```python
from build123d import *

# Parameters (mm, degrees)
ESQUISSE1_R          = 10
ESQUISSE1_R_2        = 4
BASE_EXTRUSION_DEPTH = 4
ESQUISSE2_R          = 7
ESQUISSE2_R_2        = 4
BOSS_EXTRU_1_DEPTH   = 3
CHANFREIN3_SIZE      = 0.5


with BuildPart() as part:
    # Esquisse1 → Base-Extrusion (new body)
    with BuildSketch(Plane.XY):
        Circle(ESQUISSE1_R)
        Circle(ESQUISSE1_R_2, mode=Mode.SUBTRACT)
    extrude(amount=BASE_EXTRUSION_DEPTH)

    # Esquisse2 → Boss.-Extru.1 (add)
    with BuildSketch(Plane.XY.offset(4)):
        Circle(ESQUISSE2_R)
        Circle(ESQUISSE2_R_2, mode=Mode.SUBTRACT)
    extrude(amount=BOSS_EXTRU_1_DEPTH)

    # Chanfrein3
    chanfrein3_edges = [part.edges().sort_by_distance(p)[0] for p in [
        (-7, 0, 7),
        (-4, 0, 7),
        (-4, 0, 0),
    ]]
    chamfer(chanfrein3_edges, length=CHANFREIN3_SIZE)


solid = part.part
```
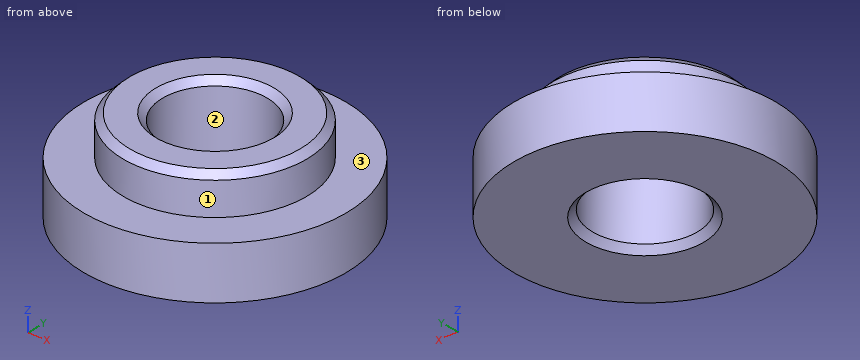
Geometry check sheet. Reference: the model listing, model coordinates, mm. Face numbers are marked on the shaded views. Coordinates: 2 decimals unless noted, no trailing zeros. Order: outer loops, then holes, each group sorted by start corner. A loop starts at its lowest first (then second) coordinate and runs counter-clockwise, first axis right, second up. Notation, with made-up numbers: (21, 11.25) - (35, 11.25) arc R24 ccw to (35, 49.25) - close; hole circle Ø7 at (-27.75, -5). An arc over 180 degrees is marked (long way). Answer as a JSON object with one key per item and string values. Group by question number.
Item 1: Sectioned sample at C-C, the plane z = 1.5. Record the cut outline in (x, y), and give its area (3 significant figures).
Item 2: Depth check by flat-ended pin: pin 1 Ø4 at (x, z) = (-5.5, 2) entering from +Y; pin 2 Ø1.5 at (y, z) = (-3, 6) entering from +X; pin 3 Ø3 at (x, z) = (-2.5, 6) entering from -Y. Enter the tip coordinate at first touch or a pass-through.
Item 3: Draft check along X on the marked faces 1, 2 and 3. Enter one of: +X half, -X half, draft (parallel to the pull), parting line (faces both ways), or undercut.
Item 4: Scan lines: probe 1 along Y at (x, z) = (0, 2.7); probe 2 along Y at (x, z) = (0, 4.65); probe 3 along Z at (x, y) = (-0.5, -8.5). Record each from-to range of solid material in increasing order.
Item 5: Sectioned sample at A-A, the plane y = 0. Record the cut outline in (x, z).
Item 6: Sectioned sample at D-D, the plane y = -8. Record the cut outline in (x, z).
Resolved:
{
 "1": {"outline": "circle Ø20 at (0, 0); hole circle Ø8 at (0, 0)", "area": "264 mm^2"},
 "2": {"pin 1": "y = 9.37", "pin 2": "x = 6.63", "pin 3": "y = -6.93"},
 "3": {"face 1": "parting line", "face 2": "undercut", "face 3": "draft"},
 "4": {"probe 1": "-10 to -4, 4 to 10", "probe 2": "-7 to -4, 4 to 7", "probe 3": "0 to 4"},
 "5": {"outline": "(-10, 0) - (-4.5, 0) - (-4, 0.5) - (-4, 6.5) - (-4.5, 7) - (-6.5, 7) - (-7, 6.5) - (-7, 4) - (-10, 4) - close; (4, 0.5) - (4.5, 0) - (10, 0) - (10, 4) - (7, 4) - (7, 6.5) - (6.5, 7) - (4.5, 7) - (4, 6.5) - close"},
 "6": {"outline": "(-6, 0) - (6, 0) - (6, 4) - (-6, 4) - close"}
}
